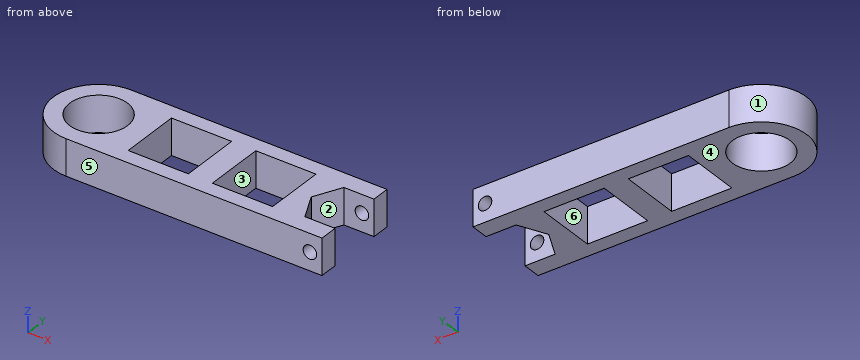
```python
from build123d import *

# Parameters (mm, degrees)
SKETCH1_R           = 9.625
BOSS_EXTRUDE1_DEPTH = 12
SKETCH2_R           = 2.25
CUT_EXTRUDE1_DEPTH  = 106.090437243
SKETCH3_W           = 20
SKETCH3_H           = 20
CUT_EXTRUDE2_DEPTH  = 102.828286836


with BuildPart() as part:
    # Sketch1 → Boss-Extrude1 (new body)
    with BuildSketch(Plane.XY):
        with BuildLine():
            Line((-85, 15), (0, 15))
            Line((0, 15), (0, 9))
            Line((0, 9), (-10, 9))
            Line((-10, 9), (-14.358898944, 0))
            Line((-14.358898944, 0), (-10, -9))
            Line((-10, -9), (0, -9))
            Line((0, -9), (0, -15))
            Line((0, -15), (-85, -15))
            ThreePointArc((-85, -15), (-100, 0), (-85, 15))
        make_face()
        with Locations((-85, 0)):
            Circle(SKETCH1_R, mode=Mode.SUBTRACT)
    extrude(amount=BOSS_EXTRUDE1_DEPTH)

    # Sketch2 → Cut-Extrude1 (cut, through all)
    with BuildSketch(Plane.XZ.offset(15)):
        with Locations((-4, 6)):
            Circle(SKETCH2_R)
    extrude(amount=-CUT_EXTRUDE1_DEPTH, mode=Mode.SUBTRACT)

    # Sketch3 → Cut-Extrude2 (cut, through all)
    with BuildSketch(Plane.XY.offset(12)):
        with Locations((-30, 0)):
            Rectangle(SKETCH3_W, SKETCH3_H)
        with Locations((-58, 0)):
            Rectangle(SKETCH3_W, SKETCH3_H)
    extrude(amount=-CUT_EXTRUDE2_DEPTH, mode=Mode.SUBTRACT)


solid = part.part
```
The model under review builds one solid part; all positions refer to its coordinate system, in mm. Face numbers are marked on the shaded views. A direction names the side the tool comes from. Give positions to 0.01 mm unless a question says otherwise; leave off trailing zeros. Write each loop counter-clockwise with the first axis right and the second up, starting at its lowest first coordinate (ties: lowest second). Pieces come first, ordered by that corner, then holes. Notation, with made-up numbers: M -27,9.5 L 27,9.5 A30 cw 27,44.5 Z; hole C 12,34 d1. An arc over 180 degrees is marked long. Answer in a Markdown table with one row per item.
Item 1: For P1, Ø6, axis at x = -79.5, y = -6.5, coming from the +Z side; P2, Ø3.5, axis at y = 2, z = 7, coming from the +X side; P3, Ø1.5, axis at y = 3, z = 3.5, coming from the -X side, all flat-tipped, find the tip position at first contact; note any pin that passes through.
Check sheet entries:
| item | result |
|---|---|
| P1 | z = 12 |
| P2 | x = -12.54 |
| P3 | x = -99.83 |
Item 2: Draft analysis for pull direction Y (two halves, no side actions). For the marked faces 4, 5 and 6, state which applies: +Y half, -Y half, draft (parallel to the pull), parting line (faces both ways), or undercut.
Check sheet entries:
| item | result |
|---|---|
| face 4 | draft |
| face 5 | -Y half |
| face 6 | undercut |
Item 3: For line 1 along Z through (x, y) = (-4, 13.6); line 2 along Y through (x, z) = (-66.5, 5.5); line 3 along Y through (x, z) = (-8.5, 4.25), list the stretches that pass through material, from the lowest coordinate up.
Check sheet entries:
| item | result |
|---|---|
| line 1 | 0 to 3.75, 8.25 to 12 |
| line 2 | -15 to -10, 10 to 15 |
| line 3 | -15 to -9, 9 to 15 |
Item 4: Add section D-D on x = -4. Give the boundary of the cut face in (y, z).
Check sheet entries:
| item | result |
|---|---|
| outline | M -15,0 L -9,0 L -9,3.75 L -15,3.75 Z; M -15,8.25 L -9,8.25 L -9,12 L -15,12 Z; M 9,0 L 15,0 L 15,3.75 L 9,3.75 Z; M 9,8.25 L 15,8.25 L 15,12 L 9,12 Z |
Item 5: Add section C-C on y = -1. Give the boundary of the cut face in (x, z), plus the area to 3 significant figures.
Check sheet entries:
| item | result |
|---|---|
| outline | M -99.97,0 L -94.57,0 L -94.57,12 L -99.97,12 Z; M -75.43,0 L -68,0 L -68,12 L -75.43,12 Z; M -48,0 L -40,0 L -40,12 L -48,12 Z; M -20,0 L -13.87,0 L -13.87,12 L -20,12 Z |
| area | 323 mm2 |
Item 6: Tool access review of the marked faces 1, 2 and 3: name each direction out of +Z, -Z, +X, -X, +Y, -Y from which nothing blocks a thin tool from reaching the whole face with its end or side.
Check sheet entries:
| item | result |
|---|---|
| face 1 | +Z, -Z, -X |
| face 2 | +Z, -Z, +X |
| face 3 | +Z, -Z |
Item 7: Add section B-B on x = -28. Give the boundary of the cut face in (y, z), plus the area to 3 significant figures.
Check sheet entries:
| item | result |
|---|---|
| outline | M -15,0 L -10,0 L -10,12 L -15,12 Z; M 10,0 L 15,0 L 15,12 L 10,12 Z |
| area | 120 mm2 |
Item 8: Add section A-A on z = 6. Give the boundary of the cut face in (x, y) (3 decimals), plus the area to 3 significant figures.
Check sheet entries:
| item | result |
|---|---|
| outline | M -85,-15 L -6.25,-15 L -6.25,-9 L -10,-9 L -14.359,0 L -10,9 L -6.25,9 L -6.25,15 L -85,15 A15 ccw Z; M -1.75,-15 L 0,-15 L 0,-9 L -1.75,-9 Z; M -1.75,9 L 0,9 L 0,15 L -1.75,15 Z; hole C -85,0 d19.25; hole M -68,-10 L -48,-10 L -48,10 L -68,10 Z; hole M -40,-10 L -20,-10 L -20,10 L -40,10 Z |
| area | 1,540 mm2 |
